For this review, take the finished solid that the model builds, in its own axes (mm). Coordinates: 2 decimals unless noted, no trailing zeros. Order: outer loops, then holes, each group sorted by start corner. A loop starts at its lowest first (then second) coordinate and runs counter-clockwise, first axis right, second up. Notation, with made-up numbers: (48, 63) -> (53, 63) arc R16 cw to (53, 94) -> close; hole circle Ø4 at (55.25, -2). An arc over 180 degrees is marked (long way). Return JSON: item names as keys, results as strings. Group by question number.
Item 1: Take a section at C-C (y = -133.5). Write out the cut boundary in (x, z).
Item 2: Take a section at D-D (y = -88). Write out the cut boundary in (x, z), then the cut area to 3 significant figures.
Item 3: Take a section at B-B (y = 60). Write out the cut boundary in (x, z).
Item 4: For line 1 along X through (y, z) = (-83.5, 5); line 2 along Y through (x, z) = (-125, 3); line 3 along X through (y, z) = (111, 2.75), list the stretches that pass through material, from the lowest coordinate up.
Item 5: Take a section at A-A (z = 6.5). Write out the cut boundary in (x, y).
Item 6: Insertion check: pin 1 (3 mm diameter, centred on y = 37.5, z = 7, fed in from -X); pin 2 (4 mm diameter, centred on y = 114, z = 3.5, fed in from +X); pin 3 (1.5 mm diameter, centred on y = -26, z = 6.5, fed in from +X); pin 4 (5 mm diameter, centred on x = 0, y = 0, fed in from +Z). Each pin has a flat end and moves straight along its axis. Give the tip position at first contact, or say it passes through.
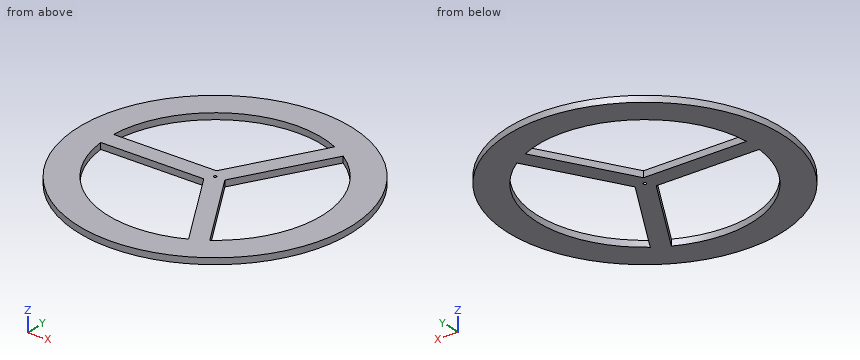
```python
from build123d import *

# Parameters (mm, degrees)
SKETCH1_R               = 175
BOSS_EXTRUDE1_DEPTH     = 8
SKETCH2_R               = 1.9
CUT_EXTRUDE2_DEPTH      = 9
CUT_EXTRUDE2_DEPTH_BACK = 1


with BuildPart() as part:
    # Sketch1 → Boss-Extrude1 (new body)
    with BuildSketch(Plane.XY):
        Circle(SKETCH1_R)
        with BuildLine():
            Line((-6.25, 10.825317547), (-137.073201247, 10.825317547))
            ThreePointArc((-137.073201247, 10.825317547), (-68.75, 119.07849302), (59.161600623, 124.121533231))
            Line((59.161600623, 124.121533231), (-6.25, 10.825317547))
        make_face(mode=Mode.SUBTRACT)
        with BuildLine():
            Line((-6.25, -10.825317547), (-137.073201247, -10.825317547))
            ThreePointArc((-137.073201247, -10.825317547), (-68.75, -119.07849302), (59.161600623, -124.121533231))
            Line((59.161600623, -124.121533231), (-6.25, -10.825317547))
        make_face(mode=Mode.SUBTRACT)
        with BuildLine():
            Line((12.5, 0), (77.911600623, 113.296215684))
            ThreePointArc((77.911600623, 113.296215684), (137.5, 0), (77.911600623, -113.296215684))
            Line((77.911600623, -113.296215684), (12.5, 0))
        make_face(mode=Mode.SUBTRACT)
    extrude(amount=BOSS_EXTRUDE1_DEPTH)

    # Sketch2 → Cut-Extrude2 (cut, two sides)
    with BuildSketch(Plane.XY) as cut_extrude2_sk:
        Circle(SKETCH2_R)
    extrude(amount=CUT_EXTRUDE2_DEPTH, mode=Mode.SUBTRACT)
    extrude(cut_extrude2_sk.sketch, amount=-CUT_EXTRUDE2_DEPTH_BACK, mode=Mode.SUBTRACT)


solid = part.part
```
Findings below:
{
 "1": {"outline": "(-113.15, 0) -> (-32.92, 0) -> (-32.92, 8) -> (-113.15, 8) -> close; (32.92, 0) -> (113.15, 0) -> (113.15, 8) -> (32.92, 8) -> close"},
 "2": {"outline": "(-151.26, 0) -> (-105.65, 0) -> (-105.65, 8) -> (-151.26, 8) -> close; (38.31, 0) -> (63.31, 0) -> (63.31, 8) -> (38.31, 8) -> close; (105.65, 0) -> (151.26, 0) -> (151.26, 8) -> (105.65, 8) -> close", "area": "930 mm2"},
 "3": {"outline": "(-164.39, 0) -> (-123.72, 0) -> (-123.72, 8) -> (-164.39, 8) -> close; (22.14, 0) -> (47.14, 0) -> (47.14, 8) -> (22.14, 8) -> close; (123.72, 0) -> (164.39, 0) -> (164.39, 8) -> (123.72, 8) -> close"},
 "4": {"line 1": "x = -153.79 to -109.24, 35.71 to 60.71, 109.24 to 153.79", "line 2": "y = -122.47 to -57.28, -10.83 to 10.83, 57.28 to 122.47", "line 3": "x = -135.29 to -81.15, 51.59 to 76.59, 81.15 to 135.29"},
 "5": {"outline": "circle Ø350 at (0, 0); hole (-137.07, -10.83) arc R137.5 ccw to (59.16, -124.12) -> (-6.25, -10.83) -> close; hole (-137.07, 10.83) -> (-6.25, 10.83) -> (59.16, 124.12) arc R137.5 ccw to start; hole circle Ø3.8 at (0, 0); hole (12.5, 0) -> (77.91, -113.3) arc R137.5 ccw to (77.91, 113.3) -> close"},
 "6": {"pin 1": "stops at x = -171.26", "pin 2": "stops at x = 134.47", "pin 3": "stops at x = 173.17", "pin 4": "stops at z = 8"}
}
